from build123d import *

# Parameters (mm, degrees)
SKETCH_3_W          = 41.5
SKETCH_3_H          = 40
EXTRUDE_1_DEPTH     = 1.5
SKETCH_4_W          = 1.5
SKETCH_4_H          = 40
EXTRUDE_2_DEPTH     = 44.5
SKETCH_5_R          = 1.75
CUT_EXTRUDE_1_DEPTH = 1.5
SKETCH_6_R          = 1.6
CUT_EXTRUDE_2_DEPTH = 1.5
FILLET_3_R          = 20
FILLET_4_R          = 3


with BuildPart() as part:
    # 草图3 → 凸台-拉伸1 (new body)
    with BuildSketch(Plane(origin=(0, 0, 0), x_dir=(1, 0, 0), z_dir=(0, 1, 0))):
        Rectangle(SKETCH_3_W, SKETCH_3_H)
    extrude(amount=EXTRUDE_1_DEPTH)

    # 草图4 → 凸台-拉伸2 (add)
    with BuildSketch(Plane(origin=(0, 1.5, 0), x_dir=(1, 0, 0), z_dir=(0, 1, 0))):
        with Locations((-20, 0)):
            Rectangle(SKETCH_4_W, SKETCH_4_H)
    extrude(amount=EXTRUDE_2_DEPTH)

    # 草图5 → 切除-拉伸1 (cut)
    with BuildSketch(Plane(origin=(0, 1.5, 0), x_dir=(1, 0, 0), z_dir=(0, 1, 0))):
        with Locations(Location((-11.25, 15, 0), (0, 0, 270))):
            Circle(SKETCH_5_R)
        with Locations(Location((12.75, 15, 0), (0, 0, 270))):
            Circle(SKETCH_5_R)
        with Locations(Location((-11.25, -15, 0), (0, 0, 270))):
            Circle(SKETCH_5_R)
        with Locations(Location((12.75, -15, 0), (0, 0, 270))):
            Circle(SKETCH_5_R)
    extrude(amount=-CUT_EXTRUDE_1_DEPTH, mode=Mode.SUBTRACT)

    # 草图6 → 切除-拉伸2 (cut)
    with BuildSketch(Plane(origin=(-19.25, 0, 0), x_dir=(0, 0, -1), z_dir=(1, 0, 0))):
        with Locations((-15.5, 26)):
            Circle(SKETCH_6_R)
        with Locations((-7.75, 39.423393759)):
            Circle(SKETCH_6_R)
        with Locations((7.75, 39.423393759)):
            Circle(SKETCH_6_R)
        with Locations((15.5, 26)):
            Circle(SKETCH_6_R)
        with Locations((7.75, 12.576606241)):
            Circle(SKETCH_6_R)
        with Locations((-7.75, 12.576606241)):
            Circle(SKETCH_6_R)
        with BuildLine():
            Line((-6.5, 33), (-6.5, 19))
            ThreePointArc((-6.5, 19), (0, 12.5), (6.5, 19))
            Line((6.5, 19), (6.5, 33))
            ThreePointArc((6.5, 33), (0, 39.5), (-6.5, 33))
        make_face()
    extrude(amount=-CUT_EXTRUDE_2_DEPTH, mode=Mode.SUBTRACT)

    # 圆角3
    fillet_3_edges = [part.edges().sort_by_distance(p)[0] for p in [
        (-20, 46, -20),
        (-20, 46, 20),
    ]]
    fillet(fillet_3_edges, radius=FILLET_3_R - 0.0001)  # a hair under: the kernel refuses the full size

    # 圆角4
    fillet_4_edges = [part.edges().sort_by_distance(p)[0] for p in [
        (20.75, 0.75, 20),
        (20.75, 0.75, -20),
    ]]
    fillet(fillet_4_edges, radius=FILLET_4_R)


solid = part.part
Verification items for the finished model (mm, model axes). A direction names the side the tool comes from. Give positions to 0.01 mm unless a question says otherwise; leave off trailing zeros. Loops run counter-clockwise (first coordinate to the right, second up) from the corner with the lowest first, then second, coordinate; pieces in that order, holes last. Notation, with made-up numbers: (-25.75, -2.75) - (3.25, -2.75) arc R29 cw to (3.25, 31.25) - close; hole circle Ø6 at (56.25, -26.5). An arc over 180 degrees is marked (long way). Write item = value, one per line. Start each with the question number.
Q1. Cross-section at B-B, the plane y = 22. Enter the section's corners in (x, z).
Q2. Depth check by flat-ended pin: P1, Ø3.5, axis at y = 39.42, z = -7.75, coming from the +X side; P2, Ø1.2, axis at x = -20, y = 27, coming from the +Z side; P3, Ø4, axis at x = -1.5, z = 7, coming from the +Y side. Enter the tip coordinate at first touch or a pass-through.
Q3. Thickness scan on line 1 (X direction, y = 0.95, z = -15); line 2 (X direction, y = 15.5, z = -11.5); line 3 (Y direction, x = -19.85, z = 7.75). Record the ranges inside material, lowest first.
Q4. Cross-section at D-D, the plane z = -15.5. Enter the section's corners in (x, y).
Q5. Cross-section at A-A, the plane x = 12.75. Enter the section's corners in (y, z), and give its area (3 significant figures).
Q6. Mould release check, pull along X, two halves, no side actions. Record for faces 1 (the face through (-9.774, 0.76, 15.941)), 2 (the face through (-7, 1, -20)), 3 (the face through (14.226, 0.76, 15.941)), 4 (the face through (-20.75, 12, 0)): released by +X, released by -X, zero draft, split by the parting line, or undercut.
Q7. Cross-section at C-C, the plane z = 7.5. Enter the section's corners in (x, y).
Q8. Tool access check on faces 5 (the face through (-19.25, 14, 5)), 6 (the face through (-20, 26, -6.5)), 7 (the face through (-19.99, 40.297, -13.986)). Record the directions out of +Z, -Z, +X, -X, +Y, -Y that give a thin tool (end or side, any length) a straight path to the whole face; none if there is none.
Answer key:
q1.outline = (-20.75, -20) - (-19.25, -20) - (-19.25, -6.5) - (-20.75, -6.5) - close; (-20.75, 6.5) - (-19.25, 6.5) - (-19.25, 20) - (-20.75, 20) - close
q2.P1 = -19.25
q2.P2 = 20
q2.P3 = 1.5
q3.line_1 = -20.75 to -13, -9.5 to 11, 14.5 to 20.75
q3.line_2 = -20.75 to -19.25
q3.line_3 = 0 to 10.98, 14.18 to 37.82, 41.02 to 44.44
q4.outline = (-20.75, 0) - (-12.93, 0) - (-12.93, 1.5) - (-19.25, 1.5) - (-19.25, 24.4) - (-20.75, 24.4) - close; (-20.75, 27.6) - (-19.25, 27.6) - (-19.25, 38.64) - (-20.75, 38.64) - close; (-9.57, 0) - (11.07, 0) - (11.07, 1.5) - (-9.57, 1.5) - close; (14.43, 0) - (20.75, 0) - (20.75, 1.5) - (14.43, 1.5) - close
q5.outline = (0, -20) - (1.5, -20) - (1.5, -16.75) - (0, -16.75) - close; (0, -13.25) - (1.5, -13.25) - (1.5, 13.25) - (0, 13.25) - close; (0, 16.75) - (1.5, 16.75) - (1.5, 20) - (0, 20) - close
q5.area = 49.5 mm^2
q6.face_1 = undercut
q6.face_2 = zero draft
q6.face_3 = undercut
q6.face_4 = released by -X
q7.outline = (-20.75, 0) - (20.75, 0) - (20.75, 1.5) - (-19.25, 1.5) - (-19.25, 11) - (-20.75, 11) - close; (-20.75, 14.16) - (-19.25, 14.16) - (-19.25, 37.84) - (-20.75, 37.84) - close; (-20.75, 41) - (-19.25, 41) - (-19.25, 44.54) - (-20.75, 44.54) - close
q8.face_5 = +Z, -Z, +X, +Y
q8.face_6 = +X, -X
q8.face_7 = -Z, +X, -X, +Y
